Geometry check sheet. Reference: the model listing, model coordinates, mm. A direction names the side the tool comes from. Give positions to 0.01 mm unless a question says otherwise; leave off trailing zeros. Write each loop counter-clockwise with the first axis right and the second up, starting at its lowest first coordinate (ties: lowest second). Pieces come first, ordered by that corner, then holes. Notation, with made-up numbers: (-20, 77) -> (33, 77) arc R15 cw to (33, 81) -> close; hole circle Ø2 at (36, -33.75). An arc over 180 degrees is marked (long way). One line per item, written item: value.
from build123d import *

# Parameters (mm, degrees)
BOSS_EXTRUDE1_DEPTH  = 3.175
MIRROR2_COPY_1_DEPTH = 3.175
SKETCH2_W            = 44.45
SKETCH2_H            = 76.2
BOSS_EXTRUDE2_DEPTH  = 3.175
CHAMFER1_SIZE        = 10


with BuildPart() as part:
    # Sketch1 → Boss-Extrude1 (new body)
    with BuildSketch(Plane.XY):
        Polygon((0, -6.997959184), (0, -0.647959184), (-22.86, -0.647959184), (-22.86, 34.912040816), (-26.67, 34.912040816), (-26.67, -6.997959184), align=None)
    boss_extrude1 = extrude(amount=BOSS_EXTRUDE1_DEPTH)

    # Mirror1: Boss-Extrude1 across plane
    add(boss_extrude1.mirror(Plane.XY))

    # Mirror2: Boss-Extrude1 across plane
    add(boss_extrude1.mirror(Plane(origin=(0, 0, 0), x_dir=(0, 0, 1), z_dir=(1, 0, 0))))

    # Mirror2 copy 1 sketch → Mirror2 copy 1 (add)
    with BuildSketch(Plane(origin=(0, 0, 0), x_dir=(-1, 0, 0), z_dir=(0, 0, -1))):
        Polygon((0, -6.997959184), (0, -0.647959184), (-22.86, -0.647959184), (-22.86, 34.912040816), (-26.67, 34.912040816), (-26.67, -6.997959184), align=None)
    extrude(amount=MIRROR2_COPY_1_DEPTH)

    # Sketch2 → Boss-Extrude2 (add)
    with BuildSketch(Plane(origin=(0, 0, 0), x_dir=(0, 0, -1), z_dir=(1, 0, 0))):
        with Locations((0, -38.747959184)):
            Rectangle(SKETCH2_W, SKETCH2_H)
    boss_extrude2 = extrude(amount=BOSS_EXTRUDE2_DEPTH)

    # Mirror3: Boss-Extrude2 across plane
    add(boss_extrude2.mirror(Plane(origin=(0, 0, 0), x_dir=(0, 0, 1), z_dir=(1, 0, 0))))

    # Chamfer1
    chamfer1_edges = [part.edges().sort_by_distance(p)[0] for p in [
        (3.175, -3.822959184, -3.175),
        (3.175, -3.822959184, 3.175),
        (-3.175, -3.822959184, -3.175),
        (-3.175, -3.822959184, 3.175),
    ]]
    chamfer(chamfer1_edges, length=CHAMFER1_SIZE)


solid = part.part
1) Sectioned sample at D-D on y = -63.5. Record the cut outline in (x, z) (3 decimals).
Verdict:
outline: (-3.175, -22.225) -> (3.175, -22.225) -> (3.175, 22.225) -> (-3.175, 22.225) -> close
2) Tool access check on faces 1 (the flat face through (-12, -6.998, 0)), 2 (the flat face through (-22.86, 17, 0)), 3 (the flat face through (12, -6.998, 0)), 4 (the flat face through (-24, 9, 3.175)), 5 (the flat face through (23.02, 9.59, 3.175)). Record the directions out of +Z, -Z, +X, -X, +Y, -Y that give a thin tool (end or side, any length) a straight path to the whole face; none if there is none.
Verdict:
face 1: +Z, -Z, -X, -Y
face 2: +Z, -Z, +Y
face 3: +Z, -Z, +X, -Y
face 4: +Z, -X, +Y, -Y
face 5: +Z, +X, +Y, -Y
3) Sectioned sample at B-B on x = 11. Record the cut outline in (y, z), plus the area to 3 significant figures.
Verdict:
outline: (-7, -5.35) -> (-0.65, -5.35) -> (-0.65, 5.35) -> (-7, 5.35) -> close
area: 67.9 mm^2
4) Scan lines: probe 1 along X at (y, z) = (30, -2.5); probe 2 along Y at (x, z) = (1.5, -5.5); probe 3 along Y at (x, z) = (17, 2.5). Record each from-to range of solid material in increasing order.
Verdict:
probe 1: -26.67 to -22.86, 22.86 to 26.67
probe 2: -76.85 to -0.65
probe 3: -7 to -0.65
5) Sectioned sample at C-C on z = -2. Record the cut outline in (x, y) (3 decimals).
Verdict:
outline: (-26.67, -6.998) -> (-3.175, -6.998) -> (-3.175, -76.848) -> (3.175, -76.848) -> (3.175, -6.998) -> (26.67, -6.998) -> (26.67, 34.912) -> (22.86, 34.912) -> (22.86, -0.648) -> (-22.86, -0.648) -> (-22.86, 34.912) -> (-26.67, 34.912) -> close
6) Sectioned sample at A-A on z = 8. Record the cut outline in (x, y) (3 decimals).
Verdict:
outline: (-8.35, -6.998) -> (-3.175, -6.998) -> (-3.175, -76.848) -> (3.175, -76.848) -> (3.175, -6.998) -> (8.35, -6.998) -> (8.35, -0.648) -> (-8.35, -0.648) -> close
7) Depth check by flat-ended pin: pin 1 Ø4 at (x, y) = (-23, 5) entering from -Z (3 decimals); pin 2 Ø13.5 at (x, z) = (9.5, 11) entering from +Y; pin 3 Ø4 at (y, z) = (-24, 1) entering from +X (3 decimals). Enter the tip coordinate at first touch or a pass-through.
Verdict:
pin 1: z = -3.175
pin 2: y = -0.65
pin 3: x = 3.175
